Read the model definition and answer for the solid it produces. Units are mm, in the model's axes. A direction names the side the tool comes from. Coordinates: 2 decimals unless noted, no trailing zeros. Order: outer loops, then holes, each group sorted by start corner. A loop starts at its lowest first (then second) coordinate and runs counter-clockwise, first axis right, second up. Notation, with made-up numbers: (-17, 43.5) - (41, 43.5) arc R27 cw to (41, 69.5) - close; hole circle Ø5 at (60, -27). An arc over 180 degrees is marked (long way). Answer as a JSON object with one key per item and string values. Group by question number.
from build123d import *

# Parameters (mm, degrees)
BOSS_EXTRUDE1_DEPTH     = 30
CUT_EXTRUDE1_DEPTH      = 74.484692283
CUT_EXTRUDE1_DEPTH_BACK = 74.484692283
SKETCH6_R               = 10.5
CUT_EXTRUDE2_DEPTH      = 52.961524285
CUT_EXTRUDE2_DEPTH_BACK = 52.961524285
SKETCH7_R               = 1.5
SKETCH8_R               = 3
CUT_EXTRUDE3_DEPTH      = 10


with BuildPart() as part:
    # Sketch5 → Boss-Extrude1 (new, symmetric)
    with BuildSketch(Plane.XY):
        with BuildLine():
            Line((15, 30), (-15, 30))
            Line((-15, 30), (-15, 14))
            ThreePointArc((-15, 14), (-17.928932188, 6.928932188), (-25, 4))
            Line((-25, 4), (-30, 4))
            Line((-30, 4), (-30, 0))
            Line((-30, 0), (30, 0))
            Line((30, 0), (30, 4))
            Line((30, 4), (25, 4))
            ThreePointArc((25, 4), (17.928932188, 6.928932188), (15, 14))
            Line((15, 14), (15, 30))
        make_face()
    extrude(amount=BOSS_EXTRUDE1_DEPTH, both=True)

    # Sketch6 → Cut-Extrude1 (cut, two sides: drawn at the far end of the back side and taken through both)
    with BuildSketch(Plane(origin=(30, 0, 0), x_dir=(0, 0, -1), z_dir=(1, 0, 0)).offset(-CUT_EXTRUDE1_DEPTH_BACK)):
        with Locations(Location((-17.5, 18, 0), (0, 0, 337.607312195))):
            Circle(SKETCH6_R)
        with Locations(Location((17.5, 18, 0), (0, 0, 337.607312195))):
            Circle(SKETCH6_R)
    extrude(amount=CUT_EXTRUDE1_DEPTH + CUT_EXTRUDE1_DEPTH_BACK, mode=Mode.SUBTRACT)

    # Sketch7 → Cut-Extrude2 (cut, two sides: drawn at the far end of the back side and taken through both)
    with BuildSketch(Plane.XZ.offset(-CUT_EXTRUDE2_DEPTH_BACK)):
        with Locations(Location((-22.5, 12, 0), (0, 0, 270))):
            Circle(SKETCH7_R)
        with Locations(Location((22.5, 12, 0), (0, 0, 270))):
            Circle(SKETCH7_R)
        with Locations(Location((22.5, -12, 0), (0, 0, 270))):
            Circle(SKETCH7_R)
        with Locations(Location((-22.5, -12, 0), (0, 0, 270))):
            Circle(SKETCH7_R)
    extrude(amount=CUT_EXTRUDE2_DEPTH + CUT_EXTRUDE2_DEPTH_BACK, mode=Mode.SUBTRACT)

    # Sketch8 → Cut-Extrude3 (cut)
    with BuildSketch(Plane(origin=(0, 4, 0), x_dir=(1, 0, 0), z_dir=(0, 1, 0))):
        with Locations((22.5, -12)):
            Circle(SKETCH8_R)
        with Locations((22.5, 12)):
            Circle(SKETCH8_R)
        with Locations((-22.5, 12)):
            Circle(SKETCH8_R)
        with Locations((-22.5, -12)):
            Circle(SKETCH8_R)
    extrude(amount=CUT_EXTRUDE3_DEPTH, mode=Mode.SUBTRACT)


solid = part.part
1. A cutting plane is placed at B-B on z = 17.5. Write down the section's boundary in (x, y), and give its area (3 significant figures).
2. Given pin 1 (7 mm diameter, centred on x = -22.5, z = 12, fed in from +Y); pin 2 (12 mm diameter, centred on y = 20.5, z = 6.5, fed in from +X); pin 3 (3 mm diameter, centred on y = 12.5, z = 8.5, fed in from +X); pin 4 (4 mm diameter, centred on x = 9, z = -5.5, fed in from -Y), each flat-ended and moving along its own axis, determine where each tip first touches the part or whether it passes through.
3. A cutting plane is placed at A-A on y = 18. Write down the section's boundary in (x, z).
4. A cutting plane is placed at D-D on x = 4. Write down the section's boundary in (y, z), and give its area (3 significant figures).
5. For a pull along Y with two mould halves and no side action, classify faces 4 (the cylindrical face through (-21.49, 2.03, 13.11)), 5 (the cylindrical face through (-0.24, 7.54, -18.43)), 6 (the cylindrical face through (-17.85, 7.01, 0.42)) as pulls with the +Y half, pulls with the -Y half, needs draft (parallel to the pull), parting line crosses it, or undercut.
6. Straight lines are drawn through the part: L1, parallel to Z at x = 22.5, y = 2.55; L2, parallel to X at y = 1.95, z = -12; L3, parallel to Y at x = -5.5, z = 17. For each, find the intervals that lie inside material, in ascending order.
7. For faces 1 (the flat face through (15, 24, 0)), 2 (the flat face through (-15, 24, 0)), 3 (the flat face through (0, 15, 30)), determine the directions among +Z, -Z, +X, -X, +Y, -Y from which every point of the face is accessible in a straight line to the end or side of a thin tool.
8. A cutting plane is placed at C-C on x = 22.5. Write down the section's boundary in (y, z).
Derived:
{
 "1": {"outline": "(-30, 0) - (30, 0) - (30, 4) - (25, 4) arc R10 cw to (17.4, 7.5) - (-17.4, 7.5) arc R10 cw to (-25, 4) - (-30, 4) - close; (-15, 28.5) - (15, 28.5) - (15, 30) - (-15, 30) - close", "area": "423 mm2"},
 "2": {"pin 1": "stops at y = 6", "pin 2": "stops at x = 15", "pin 3": "stops at x = 15.46", "pin 4": "stops at y = 0"},
 "3": {"outline": "(-15, -30) - (15, -30) - (15, -28) - (-15, -28) - close; (-15, -7) - (15, -7) - (15, 7) - (-15, 7) - close; (-15, 28) - (15, 28) - (15, 30) - (-15, 30) - close"},
 "4": {"outline": "(0, -30) - (30, -30) - (30, 30) - (0, 30) - close; hole circle Ø21 at (18, -17.5); hole circle Ø21 at (18, 17.5)", "area": "1,110 mm2"},
 "5": {"face 4": "needs draft", "face 5": "undercut", "face 6": "pulls with the +Y half"},
 "6": {"L1": "z = -30 to -13.5, -10.5 to 10.5, 13.5 to 30", "L2": "x = -30 to -24, -21 to 21, 24 to 30", "L3": "y = 0 to 7.51, 28.49 to 30"},
 "7": {"face 1": "+Z, -Z, +X, +Y", "face 2": "+Z, -Z, -X, +Y", "face 3": "+Z, +X, -X, +Y, -Y"},
 "8": {"outline": "(0, -30) - (4.32, -30) - (4.32, -15) - (4, -15) - (4, -13.5) - (0, -13.5) - close; (0, -10.5) - (4, -10.5) - (4, -9) - (4.32, -9) - (4.32, 9) - (4, 9) - (4, 10.5) - (0, 10.5) - close; (0, 13.5) - (4, 13.5) - (4, 15) - (4.32, 15) - (4.32, 30) - (0, 30) - close"}
}
